Check sheet for the modelled part. Datum: model origin and axes. Units: mm. A direction names the side the tool comes from. Round coordinates to 2 decimals unless told otherwise and drop trailing zeros. Write each loop counter-clockwise with the first axis right and the second up, starting at its lowest first coordinate (ties: lowest second). Pieces come first, ordered by that corner, then holes. Notation, with made-up numbers: (28.5, 64.25) -> (56.5, 64.25) arc R8 ccw to (56.5, 71.25) -> close; hole circle Ø8 at (-31.75, -37.75). An arc over 180 degrees is marked (long way). One line per item, written item: value.
from build123d import *

# Parameters (mm, degrees)
SKETCH_R        = 1.5
SKETCH_R_2      = 2.5
PAD_DEPTH       = 9
FILLET_R        = 3
SKETCH001_W     = 15
SKETCH001_H     = 5
POCKET_DEPTH    = 38.601
SKETCH002_R     = 2
POCKET001_DEPTH = 7.6
CHAMFER_SIZE    = 0.2
SKETCH003_R     = 2.75
POCKET002_DEPTH = 2.9


with BuildPart() as part:
    # Sketch → Pad (new body)
    with BuildSketch(Plane.XY):
        with BuildLine():
            Line((15.5, 19.3), (-15.5, 19.3))
            ThreePointArc((-15.5, 19.3), (-18.187006, 18.187006), (-19.3, 15.5))
            Line((-19.3, 15.5), (-19.3, 0))
            ThreePointArc((-19.3, 0), (-14.3, -5), (-9.3, 0))
            Line((-9.3, 11.7), (-9.3, 0))
            Line((-9.3, 11.7), (15.5, 11.7))
            ThreePointArc((15.5, 11.7), (19.3, 15.5), (15.5, 19.3))
        make_face()
        with Locations((-15.5, 15.5)):
            Circle(SKETCH_R, mode=Mode.SUBTRACT)
        with Locations((-14.3, 0)):
            Circle(SKETCH_R_2, mode=Mode.SUBTRACT)
    extrude(amount=PAD_DEPTH)

    # Fillet
    fillet_edges = [part.edges().sort_by_distance(p)[0] for p in [
        (-9.3, 11.7, 4.5),
    ]]
    fillet(fillet_edges, radius=FILLET_R)

    # Sketch001 → Pocket (cut, through all)
    with BuildSketch(Plane(origin=(-19.3, 0, 0), x_dir=(0, -1, 0), z_dir=(-1, 0, 0))):
        with Locations((-1.5, 4.5)):
            Rectangle(SKETCH001_W, SKETCH001_H)
    extrude(amount=-POCKET_DEPTH, mode=Mode.SUBTRACT)

    # Sketch002 → Pocket001 (cut)
    with BuildSketch(Plane(origin=(0, 19.3, 0), x_dir=(-1, 0, 0), z_dir=(0, 1, 0))):
        with Locations((3.183548, 4.5)):
            Circle(SKETCH002_R)
    extrude(amount=-POCKET001_DEPTH, mode=Mode.SUBTRACT)

    # Chamfer
    chamfer_edges = [part.edges().sort_by_distance(p)[0] for p in [
        (-1.183548, 19.3, 4.5),
        (-1.183548, 11.7, 4.5),
    ]]
    chamfer(chamfer_edges, length=CHAMFER_SIZE)

    # Sketch003 → Pocket002 (cut)
    with BuildSketch(Plane.XY.offset(9)):
        with Locations((-15.5, 15.5)):
            Circle(SKETCH003_R)
    extrude(amount=-POCKET002_DEPTH, mode=Mode.SUBTRACT)


solid = part.part
Item 1: Sectioned sample at B-B on z = 7.75. Enter the section's corners in (x, y), and give its area (3 significant figures).
Answer:
outline: (-19.3, 0) arc R5 ccw to (-9.3, 0) -> (-9.3, 8.7) arc R3 cw to (-6.3, 11.7) -> (15.5, 11.7) arc R3.8 ccw to (15.5, 19.3) -> (-15.5, 19.3) arc R3.8 ccw to (-19.3, 15.5) -> close; hole circle Ø5.5 at (-15.5, 15.5); hole circle Ø5 at (-14.3, 0)
area: 399 mm^2
Item 2: Thickness scan on line 1 (X direction, y = 0, z = 7.55); line 2 (Y direction, x = -15.5, z = 7.75); line 3 (X direction, y = 16, z = 5.5). Record the ranges inside material, lowest first.
Answer:
line 1: x = -19.3 to -16.8, -11.8 to -9.3
line 2: y = -4.85 to -2.19, 2.19 to 12.75, 18.25 to 19.3
line 3: x = -19.27 to -16.91, -14.09 to -4.92, -1.45 to 19.27
Item 3: Tool access check on faces 4 (the flat face through (-9.3, 4, 1)), 5 (the flat face through (-14, 14, 6.1)), 6 (the flat face through (-14, 9, 4)). Record the directions out of +Z, -Z, +X, -X, +Y, -Y that give a thin tool (end or side, any length) a straight path to the whole face; none if there is none.
Answer:
face 4: +Z, -Z, +X, -Y
face 5: +Z
face 6: +X, -X, -Y
Item 4: Sectioned sample at A-A on y = 16. Enter the section's corners in (x, z), and give its area (3 significant figures).
Answer:
outline: (-19.27, 0) -> (-16.91, 0) -> (-16.91, 6.1) -> (-18.2, 6.1) -> (-18.2, 9) -> (-19.27, 9) -> close; (-14.09, 0) -> (19.27, 0) -> (19.27, 9) -> (-12.8, 9) -> (-12.8, 6.1) -> (-14.09, 6.1) -> close; hole circle Ø4 at (-3.18, 4.5)
area: 301 mm^2
Item 5: Sectioned sample at D-D on x = 3. Enter the section's corners in (y, z).
Answer:
outline: (11.7, 0) -> (19.3, 0) -> (19.3, 9) -> (11.7, 9) -> close
Item 6: Mould release check, pull along X, two halves, no side actions. Record for faces 1 (the flat face through (4, 11.7, 4)), 2 (the cylindrical face through (-14.4, -5, 8)), 3 (the cylindrical face through (-15.858, 18.227, 7.57)): pulls with the +X half, pulls with the -X half, needs draft (parallel to the pull), parting line crosses it, or undercut.
Answer:
face 1: needs draft
face 2: parting line crosses it
face 3: undercut
Item 7: Depth check by flat-ended pin: P1, Ø2.5, axis at x = -13.5, z = 4, coming from the -Y side; P2, Ø2.5, axis at x = -15.5, y = 15.5, coming from the -Z side; P3, Ø1.6, axis at y = 2.5, z = 1.5, coming from the +X side; P4, Ø2.5, axis at x = 6, z = 3.5, coming from the -Y side. Enter the tip coordinate at first touch or a pass-through.
Answer:
P1: stops at y = 9
P2: passes through
P3: stops at x = -9.3
P4: stops at y = 11.7
Item 8: Sectioned sample at C-C on z = 1.5. Enter the section's corners in (x, y), and give its area (3 significant figures).
Answer:
outline: (-19.3, 0) arc R5 ccw to (-9.3, 0) -> (-9.3, 8.7) arc R3 cw to (-6.3, 11.7) -> (15.5, 11.7) arc R3.8 ccw to (15.5, 19.3) -> (-15.5, 19.3) arc R3.8 ccw to (-19.3, 15.5) -> close; hole circle Ø3 at (-15.5, 15.5); hole circle Ø5 at (-14.3, 0)
area: 416 mm^2
